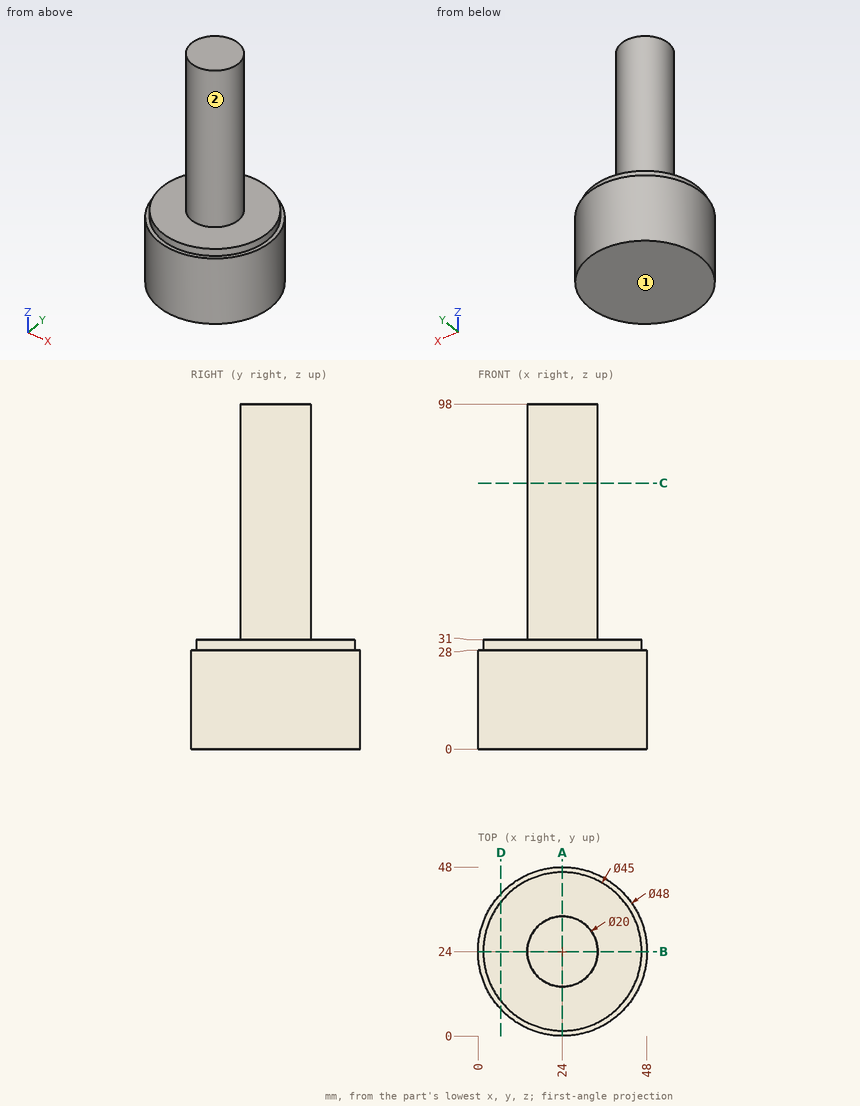
Answer from the drawing. Dimensions are ordinates in mm from the lowest x, y and z of the part. A direction names the side the tool comes from. Coordinates: 2 decimals unless noted, no trailing zeros. Write each loop counter-clockwise with the first axis right and the second up, starting at its lowest first coordinate (ties: lowest second). Pieces come first, ordered by that corner, then holes. Notation, with made-up numbers: M 73.25,-25.75 L 98.25,-25.75 A13 ccw 98.25,-1.75 Z; hole C 61,24 d5. An arc over 180 degrees is marked long. Use a Markdown table: item, result.
Q1. Each of these flat-tipped pins is pushed along its axis until it touches: pin 1 Ø8 at (x, z) = (27, 29.5) entering from +Y; pin 2 Ø1 at (x, y) = (19, 13.5) entering from +Z; pin 3 Ø4 at (y, z) = (14, 48) entering from +X. Where does it stop, or does it pass through?
Answer block:
| item | result |
|---|---|
| pin 1 | stops at y = 48 |
| pin 2 | stops at z = 31 |
| pin 3 | stops at x = 30 |
Q2. Straight lines are drawn through the part: L1, parallel to Z at x = 38.5, y = 32.5; L2, parallel to Y at x = 31, z = 79.5; L3, parallel to Y at x = 15.5, z = 81. For each, find the intervals that lie inside material, in ascending order. Write a range as [from, to].
Answer block:
| item | result |
|---|---|
| L1 | z = [0, 31] |
| L2 | y = [16.86, 31.14] |
| L3 | y = [18.73, 29.27] |
Q3. The part is cut by section A-A, the plane x = 24. Write down the section's boundary in (y, z), then the cut area to 3 significant figures.
Answer block:
| item | result |
|---|---|
| outline | M 0,0 L 48,0 L 48,28 L 46.5,28 L 46.5,31 L 34,31 L 34,98 L 14,98 L 14,31 L 1.5,31 L 1.5,28 L 0,28 Z |
| area | 2,820 mm2 |
Q4. The part is cut by section D-D, the plane x = 6.5. Write down the section's boundary in (y, z).
Answer block:
| item | result |
|---|---|
| outline | M 7.58,0 L 40.42,0 L 40.42,28 L 38.14,28 L 38.14,31 L 9.86,31 L 9.86,28 L 7.58,28 Z |
Q5. Which of the six approach directions +Z, -Z, +X, -X, +Y, -Y give full straight-line access (tool end or side, diameter ignored) to the marked faces 1 and 2?
Answer block:
| item | result |
|---|---|
| face 1 | -Z, +X, -X, +Y, -Y |
| face 2 | +Z |
Q6. The part is cut by section C-C, the plane z = 75.5. Write down the section's boundary in (x, y).
Answer block:
| item | result |
|---|---|
| outline | C 24,24 d20 |
